```python
from build123d import *

# Parameters (mm, degrees)
SKETCH_1_R          = 12.5
EXTRUDE_1_DEPTH     = 40
CHAMFER_1_SIZE      = 0.5
SKETCH_2_R          = 15
EXTRUDE_2_DEPTH     = 49
CHAMFER_2_SIZE      = 0.5
CUT_EXTRUDE_1_DEPTH = 4
SKETCH_11_R         = 14.5
EXTRUDE_3_DEPTH     = 2
SKETCH_12_R         = 20
EXTRUDE_4_DEPTH     = 1691
SKETCH_13_R         = 14.5
EXTRUDE_5_DEPTH     = 2
SKETCH_14_R         = 15
EXTRUDE_6_DEPTH     = 47
CHAMFER_3_SIZE      = 0.5


with BuildPart() as part:
    # Sketch 1 → Extrude 1 (new body)
    with BuildSketch(Plane.XY):
        Circle(SKETCH_1_R)
    extrude(amount=EXTRUDE_1_DEPTH)

    # Chamfer 1
    chamfer_1_edges = [part.edges().sort_by_distance(p)[0] for p in [
        (-12.5, 0, 40),
    ]]
    chamfer(chamfer_1_edges, length=CHAMFER_1_SIZE)

    # Sketch 2 → Extrude 2 (add)
    with BuildSketch(Plane(origin=(0, 0, 0), x_dir=(-1, 0, 0), z_dir=(0, 0, -1))):
        Circle(SKETCH_2_R)
    extrude(amount=EXTRUDE_2_DEPTH)

    # Chamfer 2
    chamfer_2_edges = [part.edges().sort_by_distance(p)[0] for p in [
        (15, 0, 0),
    ]]
    chamfer(chamfer_2_edges, length=CHAMFER_2_SIZE)

    # Sketch 5 → Cut-Extrude 1 (cut)
    with BuildSketch(Plane(origin=(0, 12.5, 0), x_dir=(1, 0, 0), z_dir=(0, 1, 0))):
        with BuildLine():
            Line((-4, -33), (-4, -11))
            ThreePointArc((-4, -11), (0, -7), (4, -11))
            Line((4, -11), (4, -33))
            ThreePointArc((4, -33), (0, -37), (-4, -33))
        make_face()
    extrude(amount=-CUT_EXTRUDE_1_DEPTH, mode=Mode.SUBTRACT)

    # Sketch 11 → Extrude 3 (add)
    with BuildSketch(Plane(origin=(0, 0, -49), x_dir=(-1, 0, 0), z_dir=(0, 0, -1))):
        Circle(SKETCH_11_R)
    extrude(amount=EXTRUDE_3_DEPTH)

    # Sketch 12 → Extrude 4 (add)
    with BuildSketch(Plane(origin=(0, 0, -51), x_dir=(-1, 0, 0), z_dir=(0, 0, -1))):
        with Locations(Location((0, 0, 0), (0, 0, 180))):
            Circle(SKETCH_12_R)
    extrude(amount=EXTRUDE_4_DEPTH)

    # Sketch 13 → Extrude 5 (add)
    with BuildSketch(Plane(origin=(0, 0, -1742), x_dir=(-1, 0, 0), z_dir=(0, 0, -1))):
        Circle(SKETCH_13_R)
    extrude(amount=EXTRUDE_5_DEPTH)

    # Sketch 14 → Extrude 6 (add)
    with BuildSketch(Plane(origin=(0, 0, -1744), x_dir=(-1, 0, 0), z_dir=(0, 0, -1))):
        Circle(SKETCH_14_R)
    extrude(amount=EXTRUDE_6_DEPTH)

    # Chamfer 3
    chamfer_3_edges = [part.edges().sort_by_distance(p)[0] for p in [
        (15, 0, -1791),
    ]]
    chamfer(chamfer_3_edges, length=CHAMFER_3_SIZE)


solid = part.part
```
Design review of the part built by this model. Coordinates are the model's own, in mm. A direction names the side the tool comes from. Give positions to 0.01 mm unless a question says otherwise; leave off trailing zeros. Write each loop counter-clockwise with the first axis right and the second up, starting at its lowest first coordinate (ties: lowest second). Pieces come first, ordered by that corner, then holes. Notation, with made-up numbers: (-19.75, 80.25) - (13.25, 80.25) arc R20 ccw to (13.25, 114.25) - close; hole circle Ø3 at (34, 84.25). An arc over 180 degrees is marked (long way). Return JSON: item names as keys, results as strings. Group by question number.
(1) To check wall thickness, follow probe 1 along Z at (x, y) = (18.5, 7); probe 2 along Y at (x, z) = (0, -1501); probe 3 along X at (y, z) = (-2.5, -662.5). State the ranges of each line that lie inside material, in increasing order.
(2) Insertion check: pin 1 (12 mm diameter, centred on x = 5.5, z = -242.5, fed in from +Y); pin 2 (3 mm diameter, centred on x = 4.5, z = -1299.5, fed in from +Y); pin 3 (9 mm diameter, centred on x = 0.5, z = 25.5, fed in from +Y). Each pin has a flat end and moves straight along its axis. Give the tip position at first contact, or say it passes through.
(3) Machinability: for faces 1 (the flat face through (11, 7, 0)), 2 (the flat face through (10.3, -10.5, -51)), 3 (the cylindrical face through (-19.98, -0.88, -884.66)), which of the approach directions +Z, -Z, +X, -X, +Y, -Y give a long, thin tool a straight path to every point of the face, cutting with its end or side? Answer none if there is none.
(4) We need section B-B, the plane z = -768.5. Give the boundary of the cut face in (x, y), then the cut area to 3 significant figures.
Reported:
{
 "1": {"probe 1": "z = -1742 to -51", "probe 2": "y = -20 to 20", "probe 3": "x = -19.84 to 19.84"},
 "2": {"pin 1": "stops at y = 20", "pin 2": "stops at y = 19.77", "pin 3": "stops at y = 11.84"},
 "3": {"face 1": "+Z", "face 2": "none", "face 3": "+Z, -Z"},
 "4": {"outline": "circle Ø40 at (0, 0)", "area": "1,260 mm2"}
}
